Geometry: see drawing. Coordinates: mm, zero at the bounding-box minimum. A direction names the side the tool comes from. Round coordinates to 2 decimals unless told otherwise and drop trailing zeros. Write each loop counter-clockwise with the first axis right and the second up, starting at its lowest first coordinate (ties: lowest second). Pieces come first, ordered by that corner, then holes. Notation, with made-up numbers: M 43,14.25 L 52,14.25 A25 cw 52,43.25 Z; hole C -34.75,34.5 d9. An arc over 180 degrees is marked long. Use one line per item in the form item = value. Start each with the question number.
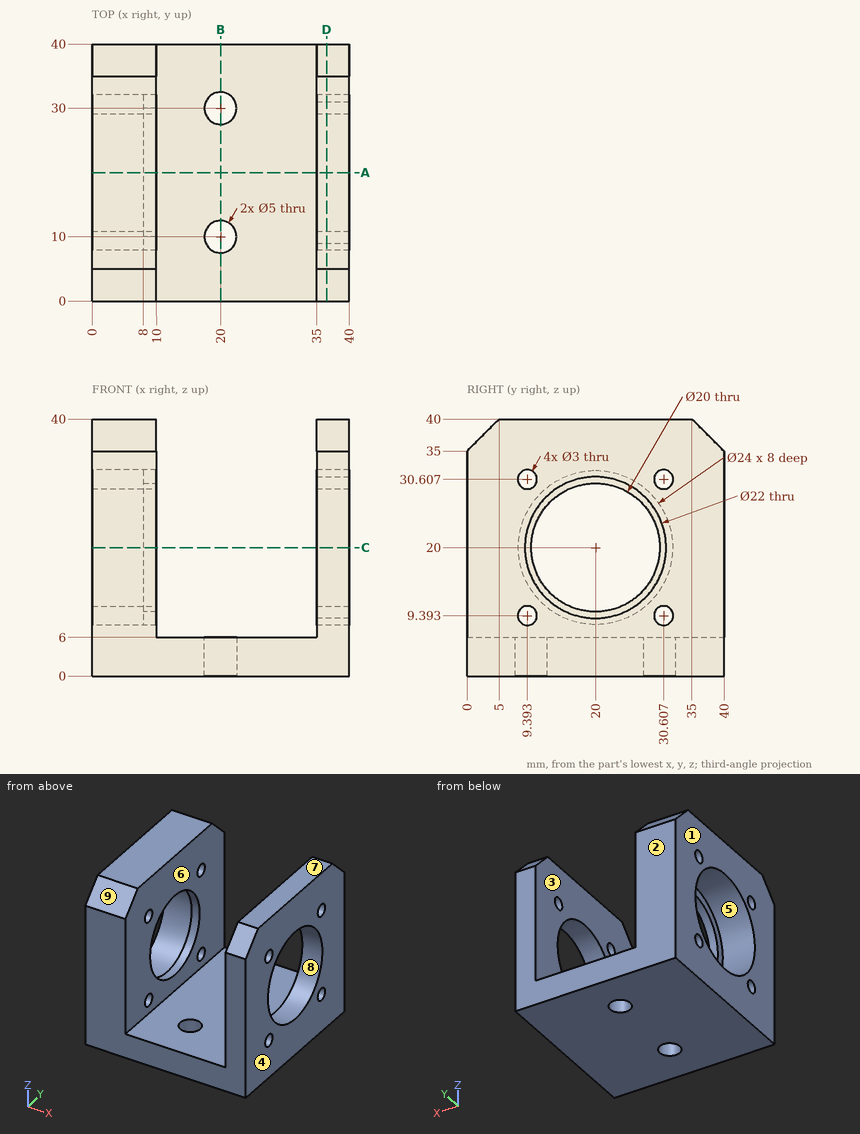
Item 1: Cut plane B-B (x = 20). Output: boundary loops of the cut face in (y, z).
Item 2: Draft query along X for the marked faces 1, 2, 3 and 4. Return one class per face: +X half, -X half, draft (parallel to the pull), parting line (faces both ways), or undercut.
Item 3: Cut plane D-D (x = 36.5). Output: boundary loops of the cut face in (y, z), plus the area to 3 significant figures.
Item 4: Cut plane C-C (z = 20). Output: boundary loops of the cut face in (x, y).
Item 5: Reachability of the marked faces 5, 6, 7, 8 and 9 from +Z, -Z, +X, -X, +Y, -Y: full face, straight path, thin tool, end or side. Return the list, or none.
Item 6: Cut plane A-A (y = 20). Output: boundary loops of the cut face in (x, z).
Item 7: Ray query, line 1 (Y direction, x = 20, z = 1.3); line 2 (X direction, y = 38, z = 24); line 3 (Z direction, x = 16.5, y = 31). Return the intervals inside material, ascending. Write a range as from..to.
Item 8: First-contact query: pin 1 (6 mm diameter, centred on x = 15, y = 30, fed in from +Z). Flat tip, straight axial feed; report the tip coordinate or a pass-through.
Final values:
q1.outline = M 0,0 L 7.5,0 L 7.5,6 L 0,6 Z; M 12.5,0 L 27.5,0 L 27.5,6 L 12.5,6 Z; M 32.5,0 L 40,0 L 40,6 L 32.5,6 Z
q2.face_1 = -X half
q2.face_2 = draft
q2.face_3 = undercut
q2.face_4 = +X half
q3.outline = M 0,0 L 40,0 L 40,35 L 35,40 L 5,40 L 0,35 Z; hole C 9.39,9.39 d3; hole C 9.39,30.61 d3; hole C 20,20 d22; hole C 30.61,9.39 d3; hole C 30.61,30.61 d3
q3.area = 1,170 mm^2
q4.outline = M 0,0 L 10,0 L 10,10 L 8,10 L 8,8 L 0,8 Z; M 0,32 L 8,32 L 8,30 L 10,30 L 10,40 L 0,40 Z; M 35,0 L 40,0 L 40,9 L 35,9 Z; M 35,31 L 40,31 L 40,40 L 35,40 Z
q5.face_5 = -X
q5.face_6 = +Z, +Y, -Y
q5.face_7 = +Z, +X, -X, +Y, -Y
q5.face_8 = +X
q5.face_9 = +Z, +X, -X, -Y
q6.outline = M 0,0 L 40,0 L 40,9 L 35,9 L 35,6 L 10,6 L 10,10 L 8,10 L 8,8 L 0,8 Z; M 0,32 L 8,32 L 8,30 L 10,30 L 10,40 L 0,40 Z; M 35,31 L 40,31 L 40,40 L 35,40 Z
q7.line_1 = 0..7.5, 12.5..27.5, 32.5..40
q7.line_2 = 0..10, 35..40
q7.line_3 = 0..6
q8.pin_1 = 6
